Source: CAD feature listing. Evaluate the final solid. Frame: model axes, mm. Coordinates: 2 decimals unless noted, no trailing zeros. Order: outer loops, then holes, each group sorted by start corner. A loop starts at its lowest first (then second) coordinate and runs counter-clockwise, first axis right, second up. Notation, with made-up numbers: (31.5, 84) -> (44.5, 84) arc R26 cw to (44.5, 120) -> close; hole circle Ø9 at (28, 50). An arc over 180 degrees is marked (long way). Put each result on its own line as item: value.
from build123d import *

# Parameters (mm, degrees)
EXTRUDE_1_DEPTH = 8


with BuildPart() as part:
    # 草图1 → 凸台-拉伸1 (new body)
    with BuildSketch(Plane.XY):
        with BuildLine():
            Line((-2.43e-07, -1.66e-07), (453.540462303, -1.66e-07))
            add(Edge.make_bspline(
                [(453.540462303, -1.66e-07), (460.79014459, 4.210016878), (469.569935404, 12.072340183), (483.622239053, 25.284804164), (493.197401943, 36.434132834), (502.695793901, 49.189345623), (511.206090033, 65.729365299), (516.029726356, 79.831331018), (518.53173017, 89.679905798)],
                knots=[0, 0, 0, 0, 0.219529356, 0.311377144, 0.509994522, 0.607272861, 0.731274185, 1, 1, 1, 1], degree=3))
            Line((518.53173017, 89.679905798), (506.162046562, 89.142399996))
            Line((506.162046562, 89.142399996), (506.162046562, 80.419495843))
            Line((506.162046562, 80.419495843), (498.162046562, 80.419495843))
            Line((498.162046562, 80.419495843), (498.162046562, 88.764379516))
            Line((498.162046562, 88.764379516), (487.370707866, 88.295458294))
            Line((487.370707866, 88.295458294), (487.370707866, 53.957597962))
            Line((487.370707866, 53.957597962), (477.370707866, 53.957597962))
            Line((477.370707866, 53.957597962), (477.370707866, 100.436233428))
            Line((477.370707866, 100.436233428), (460.65154086, 94.876216939))
            Line((460.65154086, 94.876216939), (460.65154086, 53.957597679))
            Line((460.65154086, 53.957597679), (456.65154086, 53.957597679))
            Line((456.65154086, 53.957597679), (456.65154086, 121.15189914))
            Line((456.65154086, 121.15189914), (436.824501135, 118.046777247))
            Line((436.824501135, 118.046777247), (436.824501135, 53.44350708))
            Line((436.824501135, 53.44350708), (432.824501135, 53.44350708))
            Line((432.824501135, 53.44350708), (432.824501135, 117.420335391))
            Line((432.824501135, 117.420335391), (407.629534965, 113.474540047))
            Line((407.629534965, 113.474540047), (407.629534965, 9.833214458))
            Line((407.629534965, 9.833214458), (399.629534965, 9.833214458))
            Line((399.629534965, 9.833214458), (399.629534965, 21.78896428))
            Line((399.629534965, 21.78896428), (371.149712291, 21.78896428))
            Line((371.149712291, 21.78896428), (371.149712291, 9.833214458))
            Line((371.149712291, 9.833214458), (363.149712291, 9.833214458))
            Line((363.149712291, 9.833214458), (363.149712291, 21.78896428))
            Line((363.149712291, 21.78896428), (317.013742993, 21.78896428))
            Line((317.013742993, 21.78896428), (317.013742993, 9.833214458))
            Line((317.013742993, 9.833214458), (309.013742993, 9.833214458))
            Line((309.013742993, 9.833214458), (309.013742993, 21.78896428))
            Line((309.013742993, 21.78896428), (263.112020096, 21.78896428))
            Line((263.112020096, 21.78896428), (263.112020096, 9.833214458))
            Line((263.112020096, 9.833214458), (255.112020096, 9.833214458))
            Line((255.112020096, 9.833214458), (255.112020096, 21.78896428))
            Line((255.112020096, 21.78896428), (211.237889646, 21.78896428))
            Line((211.237889646, 21.78896428), (211.237889646, 9.833214458))
            Line((211.237889646, 9.833214458), (203.237889646, 9.833214458))
            Line((203.237889646, 9.833214458), (203.237889646, 21.78896428))
            Line((203.237889646, 21.78896428), (185.170557109, 21.78896428))
            Line((185.170557109, 21.78896428), (185.170557109, 9.833214458))
            Line((185.170557109, 9.833214458), (177.170557109, 9.833214458))
            Line((177.170557109, 9.833214458), (177.170557109, 21.788961022))
            Line((177.170557109, 21.788961022), (149.785514419, 21.788961022))
            Line((149.785514419, 21.788961022), (149.785514419, 9.8332112))
            Line((149.785514419, 9.8332112), (141.785514419, 9.8332112))
            Line((141.785514419, 9.8332112), (141.785514419, 21.788961022))
            Line((141.785514419, 21.788961022), (87.128628071, 21.788961022))
            Line((87.128628071, 21.788961022), (87.128628071, 9.8332112))
            Line((87.128628071, 9.8332112), (79.128628071, 9.8332112))
            Line((79.128628071, 9.8332112), (79.128628071, 52.776041795))
            Line((79.128628071, 52.776041795), (74.39423211, 52.776041795))
            Line((74.39423211, 52.776041795), (74.39423211, 99.922139289))
            Line((74.39423211, 99.922139289), (36.732316161, 104.912244585))
            Line((36.732316161, 104.912244585), (36.732316161, 42.164639479))
            Line((36.732316161, 42.164639479), (32.732316161, 42.164639479))
            Line((32.732316161, 42.164639479), (32.732316161, 53.588490785))
            Line((32.732316161, 53.588490785), (27.905397524, 53.588490785))
            Line((27.905397524, 53.588490785), (27.905397524, 105.722742646))
            Line((27.905397524, 105.722742646), (6.037252299, 108.620214656))
            Line((6.037252299, 108.620214656), (6.037252299, 66.502939453))
            Line((6.037252299, 66.502939453), (2.037252299, 66.502939453))
            Line((2.037252299, 66.502939453), (2.037252299, 108.620214656))
            Line((2.037252299, 108.620214656), (-15.79290681, 110.982664073))
            Line((-15.79290681, 110.982664073), (-15.79290681, 103.648933932))
            Line((-15.79290681, 103.648933932), (-19.79290681, 103.648933932))
            Line((-19.79290681, 103.648933932), (-19.79290681, 110.982664073))
            Line((-19.79290681, 110.982664073), (-39.660668521, 113.615090503))
            Line((-39.660668521, 113.615090503), (-39.660668521, 104.769973164))
            Line((-39.660668521, 104.769973164), (-43.660668521, 104.769973164))
            Line((-43.660668521, 104.769973164), (-43.660668521, 113.615090503))
            Line((-43.660668521, 113.615090503), (-54.444933748, 115.043977421))
            Line((-54.444933748, 115.043977421), (-52.708792967, 109.575431))
            Line((-52.708792967, 109.575431), (-61.468269832, 106.794493648))
            Line((-61.468269832, 106.794493648), (-57.779206202, 95.174574379))
            Line((-57.779206202, 95.174574379), (-34.676393157, 87.040279865))
            Line((-34.676393157, 87.040279865), (-35.752643056, 91.631850135))
            Line((-35.752643056, 91.631850135), (-21.020693304, 89.679905349))
            Line((-21.020693304, 89.679905349), (-2.43e-07, -1.66e-07))
        make_face()
    extrude(amount=EXTRUDE_1_DEPTH)


solid = part.part
1. Ray query, line 1 along Y through (x, z) = (347.5, 7.5); line 2 along Y through (x, z) = (80.5, 4.75); line 3 along X through (y, z) = (47, 5.25). Return the intervals inside material, ascending.
Numbers:
line 1: y = 0 to 21.79
line 2: y = 0 to 9.83
line 3: x = -11.02 to 32.73, 36.73 to 79.13, 407.63 to 500.87
2. First-contact query: pin 1 (2.5 mm diameter, centred on y = 90, z = 3, fed in from +X); pin 2 (1.2 mm diameter, centred on x = -42.5, z = 4, fed in from +Y); pin 3 (4 mm diameter, centred on y = 72.5, z = 2.5, fed in from -X). Flat tips, straight axial feed; report the tip coordinate or a pass-through.
Numbers:
pin 1: stops at x = 518.53
pin 2: stops at y = 104.77
pin 3: stops at x = -17.46
3. Cut plane A-A on x = 237.5. Output: boundary loops of the cut face in (y, z).
Numbers:
outline: (0, 0) -> (21.79, 0) -> (21.79, 8) -> (0, 8) -> close
